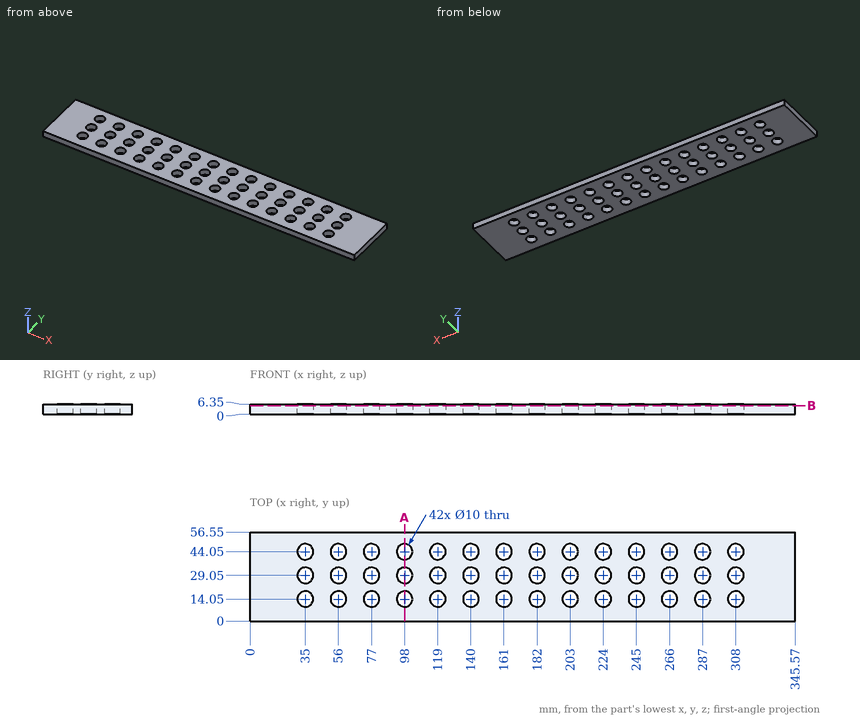
Part print with two shaded views. Sizes in mm from the minimum x, y, z corner. Coordinates: 2 decimals unless noted, no trailing zeros. Loops run counter-clockwise (first coordinate to the right, second up) from the corner with the lowest first, then second, coordinate; pieces in that order, holes last. Notation, with made-up numbers: (61, 39.25) -> (116, 39.25) arc R14 cw to (116, 56.25) -> close; hole circle Ø5 at (16.5, 36). An arc over 180 degrees is marked (long way). Answer as a JSON object with one key per item and string values.
Q1. Cut at B-B (z = 5.25). State how many separate pieces and enclosed holes the cut face has, and give its area (3 significant figures).
Report:
{"separate pieces": "1", "enclosed holes": "42", "area": "16,200 mm2"}
Q2. Probe probe 1 along Y at (x, z) = (266, 1.5); probe 2 along Y at (x, z) = (38.5, 4.5). List the from-to ranges inside material, lowest first.
Report:
{"probe 1": "y = 0 to 9.05, 19.05 to 24.05, 34.05 to 39.05, 49.05 to 56.55", "probe 2": "y = 0 to 10.48, 17.62 to 25.48, 32.62 to 40.48, 47.62 to 56.55"}
Q3. Flat gauge pin, fed straight in: P1, Ø8, axis at x = 287, y = 44.05, coming from the +Z side. Where does the tip first touch, or does it go through?
Report:
{"P1": "passes through"}
Q4. Cut at A-A (x = 98). List the corners of the cut face in (y, z), and give its area (3 significant figures).
Report:
{"outline": "(0, 0) -> (9.05, 0) -> (9.05, 6.35) -> (0, 6.35) -> close; (19.05, 0) -> (24.05, 0) -> (24.05, 6.35) -> (19.05, 6.35) -> close; (34.05, 0) -> (39.05, 0) -> (39.05, 6.35) -> (34.05, 6.35) -> close; (49.05, 0) -> (56.55, 0) -> (56.55, 6.35) -> (49.05, 6.35) -> close", "area": "169 mm2"}
